The listing builds one solid part. Answer for the finished solid, in the listing's coordinates (mm). A direction names the side the tool comes from. Round coordinates to 2 decimals unless told otherwise and drop trailing zeros. Loops run counter-clockwise (first coordinate to the right, second up) from the corner with the lowest first, then second, coordinate; pieces in that order, holes last. Notation, with made-up numbers: M 44.5,50 L 93.5,50 A14 cw 93.5,57 Z; hole C 59,71 d3. An arc over 180 degrees is marked long. Answer as a JSON object with one key per item and string values.
```python
from build123d import *

# Parameters (mm, degrees)
SKETCH_1_R      = 1.55
SKETCH_1_W      = 6.1
SKETCH_1_H      = 10
SKETCH_1_H_2    = 15.1
SKETCH_1_W_2    = 10
SKETCH_1_H_3    = 6.1
SKETCH_1_W_3    = 15
EXTRUDE_1_DEPTH = 6


with BuildPart() as part:
    # Эскиз1 → Бобышка-Вытянуть1 (new body)
    with BuildSketch(Plane(origin=(0, 0, 0), x_dir=(1, 0, 0), z_dir=(0, 1, 0))):
        with BuildLine():
            Line((-35.752327672, -33.813906094), (16.247672328, -33.813906094))
            ThreePointArc((16.247672328, -33.813906094), (19.076099452, -32.642333219), (20.247672328, -29.813906094))
            Line((20.247672328, -29.813906094), (20.247672328, 36.186093906))
            Line((20.247672328, 36.186093906), (-26.752327672, 36.186093906))
            ThreePointArc((-26.752327672, 36.186093906), (-29.580754797, 35.014521031), (-30.752327672, 32.186093906))
            Line((-30.752327672, 32.186093906), (-30.752327672, 2.186093906))
            ThreePointArc((-30.752327672, 2.186093906), (-32.698441142, -5.954712398), (-38.115964036, -12.335192834))
            ThreePointArc((-38.115964036, -12.335192834), (-39.319858012, -13.753077376), (-39.752327672, -15.562145443))
            Line((-39.752327672, -15.562145443), (-39.752327672, -29.813906094))
            ThreePointArc((-39.752327672, -29.813906094), (-38.580754797, -32.642333219), (-35.752327672, -33.813906094))
        make_face()
        with Locations((15.247672328, 2.186093906)):
            Circle(SKETCH_1_R, mode=Mode.SUBTRACT)
        with Locations((-18.752327672, -17.813906094)):
            Circle(SKETCH_1_R, mode=Mode.SUBTRACT)
        with Locations((-33.752327672, -26.813906094)):
            Circle(SKETCH_1_R, mode=Mode.SUBTRACT)
        with Locations((-18.752327672, 22.186093906)):
            Circle(SKETCH_1_R, mode=Mode.SUBTRACT)
        with Locations((15.197672328, 11.186093906)):
            Rectangle(SKETCH_1_W, SKETCH_1_H, mode=Mode.SUBTRACT)
        with Locations((-18.802327672, 2.186093906)):
            Rectangle(SKETCH_1_W, SKETCH_1_H_2, mode=Mode.SUBTRACT)
        with Locations((-1.752327672, 2.186093906)):
            Rectangle(SKETCH_1_W_2, SKETCH_1_H_3, mode=Mode.SUBTRACT)
        with Locations((15.197672328, -6.813906094)):
            Rectangle(SKETCH_1_W, SKETCH_1_H, mode=Mode.SUBTRACT)
        with Locations((1.247672328, 31.186093906)):
            Rectangle(SKETCH_1_W_3, SKETCH_1_H_3, mode=Mode.SUBTRACT)
        with Locations((1.247672328, -26.813906094)):
            Rectangle(SKETCH_1_W_3, SKETCH_1_H_3, mode=Mode.SUBTRACT)
    extrude(amount=EXTRUDE_1_DEPTH)


solid = part.part
```
Item 1: The part is cut by section A-A (z = 8). Give the vertices of the cut face in (x, y), then the cut area to 3 significant figures.
Values follow:
{"outline": "M -33.91,0 L 12.15,0 L 12.15,6 L -33.91,6 Z; M 18.25,0 L 20.25,0 L 20.25,6 L 18.25,6 Z", "area": "288 mm^2"}
Item 2: The part is cut by section D-D (y = 4.2). Give the number of separate pieces and of enclosed holes in the cut face, then the cut area to 3 significant figures.
Values follow:
{"separate pieces": "1", "enclosed holes": "10", "area": "3,300 mm^2"}
Item 3: Which of the six approach directions +Z, -Z, +X, -X, +Y, -Y give full straight-line access (tool end or side, diameter ignored) to faces 1 (the face through (-10, 3, 33.814)), 2 (the face through (12.148, 3, 7))?
Values follow:
{"face 1": "+Z, +X, -X, +Y, -Y", "face 2": "+Y, -Y"}
Item 4: Determine the mould class of faces 3 (the face through (-38.61, 2.96, 32.61)), 4 (the face through (-6.252, 3, 27)), 5 (the face through (-39.752, 3, 23)), 6 (the face through (-39.31, 2.96, 13.73)) for opening direction Z: released by +Z, released by -Z, zero draft, split by the parting line, or undercut.
Values follow:
{"face 3": "released by +Z", "face 4": "undercut", "face 5": "zero draft", "face 6": "released by -Z"}
Item 5: A flat-ended cylindrical pin translates along its axis: P1, Ø3, axis at y = 4, z = -3, coming from the -X side. Find the tip coordinate at first contact, or state that the pin passes through.
Values follow:
{"P1": "x = -30.77"}
Item 6: The part is cut by section B-B (x = -4). Give the vertices of the cut face in (y, z), then the cut area to 3 significant figures.
Values follow:
{"outline": "M 0,-36.19 L 6,-36.19 L 6,-34.24 L 0,-34.24 Z; M 0,-28.14 L 6,-28.14 L 6,-5.24 L 0,-5.24 Z; M 0,0.86 L 6,0.86 L 6,23.76 L 0,23.76 Z; M 0,29.86 L 6,29.86 L 6,33.81 L 0,33.81 Z", "area": "310 mm^2"}
Item 7: The part is cut by section C-C (x = -33.5). Give the vertices of the cut face in (y, z), then the cut area to 3 significant figures.
Values follow:
{"outline": "M 0,7.37 L 6,7.37 L 6,25.28 L 0,25.28 Z; M 0,28.34 L 6,28.34 L 6,33.81 L 0,33.81 Z", "area": "140 mm^2"}
Item 8: Straight lines are drawn through the part: line 1 (Z direction, x = 5, y = 2); line 2 (X direction, y = 3.3, z = -8); line 3 (Z direction, x = 13, y = 4). For each, find the intervals that lie inside material, in ascending order.
Values follow:
{"line 1": "-36.19 to -34.24, -28.14 to 23.76, 29.86 to 33.81", "line 2": "-30.75 to -21.85, -15.75 to 12.15, 18.25 to 20.25", "line 3": "-36.19 to -16.19, -6.19 to 1.81, 11.81 to 33.81"}
